Design review of the part built by this model. Coordinates are the model's own, in mm. Face numbers are marked on the shaded views. Give positions to 0.01 mm unless a question says otherwise; leave off trailing zeros. Write each loop counter-clockwise with the first axis right and the second up, starting at its lowest first coordinate (ties: lowest second). Pieces come first, ordered by that corner, then holes. Notation, with made-up numbers: M 59,-18.75 L 108,-18.75 A26 cw 108,19.25 Z; hole C -39.75,6 d4. An arc over 180 degrees is marked long. Answer in a Markdown table with one row per item.
```python
from build123d import *

# Parameters (mm, degrees)
CYLINDER003_R          = 1.25
CYLINDER003_DEPTH      = 8
CYLINDER003_ROLL_ANGLE = -90
CYLINDER002_R          = 5.5
CYLINDER002_DEPTH      = 8
CYLINDER002_ROLL_ANGLE = -90


with BuildPart() as m3_tap_hole:
    # Cylinder003 → Cylinder003 (new body)
    with BuildSketch(Plane.XY):
        Circle(CYLINDER003_R)
    extrude(amount=CYLINDER003_DEPTH)


with BuildPart() as m3_tap_hole_1:
    # Cylinder003 roll: moved
    add(m3_tap_hole.part.rotate(Axis((0, 0, 0), (1, 0, 0)), CYLINDER003_ROLL_ANGLE))


with BuildPart() as m3_tap_hole_2:
    # Cylinder003 placement: moved
    add(m3_tap_hole_1.part.moved(Location((17.5, 0, 6))))


with BuildPart() as m3_support_and_tap_hole:
    # Cylinder002 → Cylinder002 (new body)
    with BuildSketch(Plane.XY):
        Circle(CYLINDER002_R)
    extrude(amount=CYLINDER002_DEPTH)


with BuildPart() as m3_support_and_tap_hole_1:
    # Cylinder002 roll: moved
    add(m3_support_and_tap_hole.part.rotate(Axis((0, 0, 0), (1, 0, 0)), CYLINDER002_ROLL_ANGLE))


with BuildPart() as m3_support_and_tap_hole_2:
    # Cylinder002 placement: moved
    add(m3_support_and_tap_hole_1.part.moved(Location((17.5, 0, 6))))

    # Cut001: cut M3_tap_hole
    add(m3_tap_hole_2.part, mode=Mode.SUBTRACT)


solid = m3_support_and_tap_hole_2.part
```
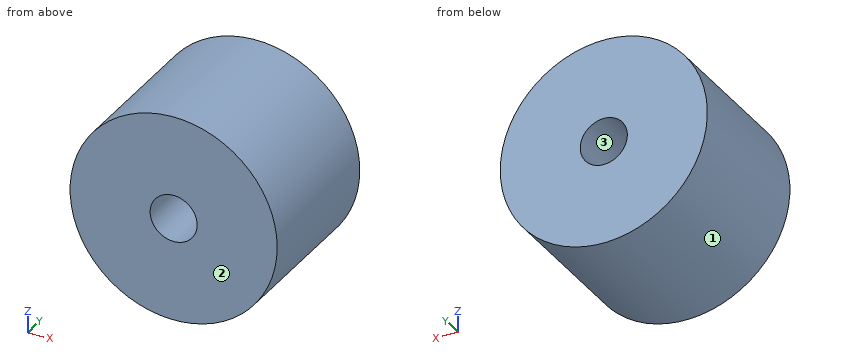
1) Insertion check: P1, Ø1.5, axis at x = 16, y = 4.5, coming from the +Z side; P2, Ø3, axis at y = 1, z = 4, coming from the -X side; P3, Ø4, axis at y = 3, z = 3, coming from the -X side. Each pin has a flat end and moves straight along its axis. Give the tip position at first contact, or say it passes through.
Geometry says:
| item | result |
|---|---|
| P1 | z = 11.45 |
| P2 | x = 12.02 |
| P3 | x = 12.09 |
2) Add section A-A (x = 17.5). Write out the cut boundary in (y, z).
Geometry says:
| item | result |
|---|---|
| outline | M 0,0.5 L 8,0.5 L 8,4.75 L 0,4.75 Z; M 0,7.25 L 8,7.25 L 8,11.5 L 0,11.5 Z |
3) Add section B-B (z = 6). Write out the cut boundary in (x, y), and give its area (3 significant figures).
Geometry says:
| item | result |
|---|---|
| outline | M 12,0 L 16.25,0 L 16.25,8 L 12,8 Z; M 18.75,0 L 23,0 L 23,8 L 18.75,8 Z |
| area | 68.0 mm^2 |
4) The part is to be moulded in two halves that separate along Z. For the marked faces 1, 2 and 3, say which applies: released by +Z, released by -Z, zero draft, split by the parting line, or undercut.
Geometry says:
| item | result |
|---|---|
| face 1 | split by the parting line |
| face 2 | zero draft |
| face 3 | undercut |
5) To check wall thickness, follow probe 1 along X at (y, z) = (6, 6); probe 2 along Z at (x, y) = (17.5, 3.75); probe 3 along X at (y, z) = (4.5, 7). State the ranges of each line that lie inside material, in increasing order. Write a range as [from, to].
Geometry says:
| item | result |
|---|---|
| probe 1 | [12, 16.25], [18.75, 23] |
| probe 2 | [0.5, 4.75], [7.25, 11.5] |
| probe 3 | [12.09, 16.75], [18.25, 22.91] |
6) Add section D-D (z = 10). Write out the cut boundary in (x, y), and give its area (3 significant figures).
Geometry says:
| item | result |
|---|---|
| outline | M 13.73,0 L 21.27,0 L 21.27,8 L 13.73,8 Z |
| area | 60.4 mm^2 |
7) Add section C-C (y = 6.75). Write out the cut boundary in (x, z).
Geometry says:
| item | result |
|---|---|
| outline | C 17.5,6 d11; hole C 17.5,6 d2.5 |
